Geometry: see drawing. Coordinates: mm, zero at the bounding-box minimum. A direction names the side the tool comes from. Round coordinates to 2 decimals unless told otherwise and drop trailing zeros. Write each loop counter-clockwise with the first axis right and the second up, starting at its lowest first coordinate (ties: lowest second). Pieces come first, ordered by that corner, then holes. Notation, with made-up numbers: (49.5, 26.5) -> (56.5, 26.5) arc R17 ccw to (56.5, 45.5) -> close; hole circle Ø4 at (0.25, 43). An arc over 180 degrees is marked (long way). Write item = value, one per line.
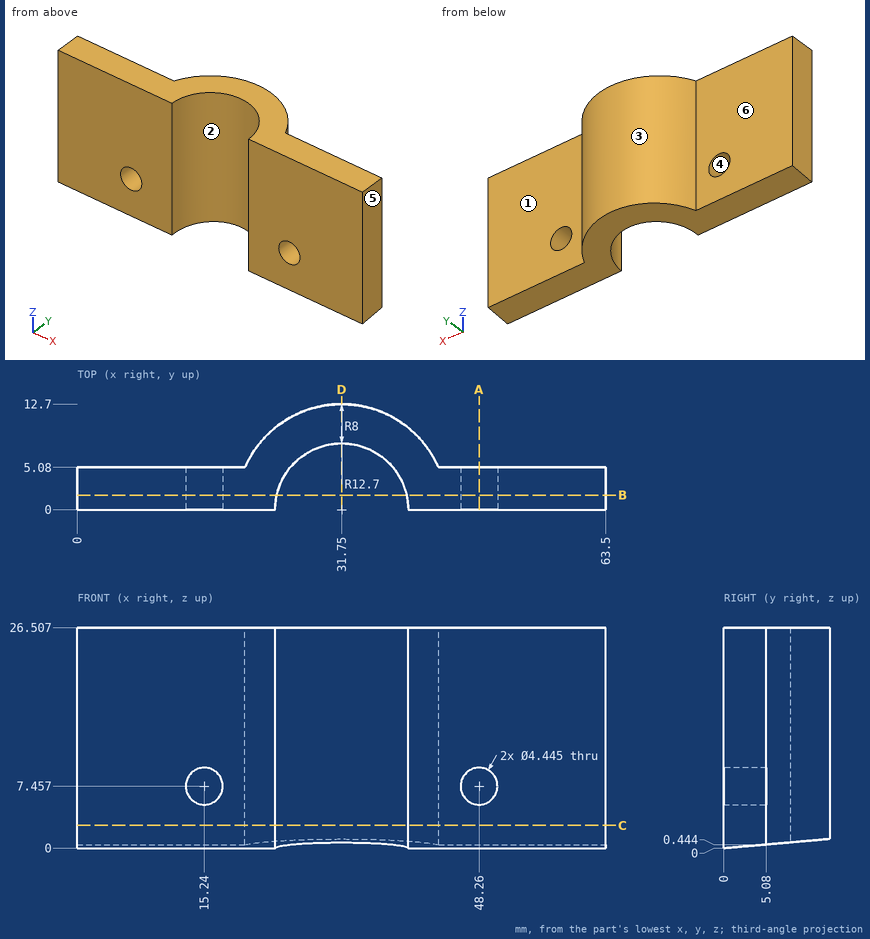
1) Cut plane D-D (x = 31.75). Return the cut outline in (y, z), and give its area (3 significant figures).
Solutions:
outline = (8, 0.7) -> (12.7, 1.11) -> (12.7, 26.51) -> (8, 26.51) -> close
area = 120 mm^2
2) Cut plane B-B (y = 1.75). Return the cut outline in (x, z) (1 decimal).
Solutions:
outline = (0, 0.2) -> (23.9, 0.2) -> (23.9, 26.5) -> (0, 26.5) -> close; (39.6, 0.2) -> (63.5, 0.2) -> (63.5, 26.5) -> (39.6, 26.5) -> close; hole circle Ø4.4 at (15.2, 7.5); hole circle Ø4.4 at (48.3, 7.5)
3) Access query for the marked faces 5 and 6. Directions: +Z, -Z, +X, -X, +Y, -Y. A direction counts if a zero-diameter tool reaches every point of the face in a straight line with its end or side. Return the directions, or none.
Solutions:
face_5 = +Z, -Z, +X, +Y, -Y
face_6 = +Z, -Z, -X, +Y
4) Cut plane C-C (z = 2.75). Return the cut outline in (x, y), and give its area (3 significant figures).
Solutions:
outline = (0, 0) -> (23.75, 0) arc R8 cw to (39.75, 0) -> (63.5, 0) -> (63.5, 5.08) -> (43.39, 5.08) arc R12.7 ccw to (20.11, 5.08) -> (0, 5.08) -> close
area = 350 mm^2
5) Cut plane A-A (x = 48.26). Return the cut outline in (y, z) (1 decimal).
Solutions:
outline = (0, 0) -> (5.1, 0.4) -> (5.1, 5.2) -> (0, 5.2) -> close; (0, 9.7) -> (5.1, 9.7) -> (5.1, 26.5) -> (0, 26.5) -> close
6) Draft query along X for the marked faces 1, 2, 3 and 4. Return one class per face: +X half, -X half, draft (parallel to the pull), parting line (faces both ways), or undercut.
Solutions:
face_1 = draft
face_2 = undercut
face_3 = parting line
face_4 = undercut
7) First-contact query: P1, Ø10, axis at x = 53.5, z = 16.5, coming from the +Y side; P2, Ø4, axis at x = 48.26, z = 7.46, coming from the -Y side; P3, Ø6, axis at y = 9.5, z = 10, coming from the -X side. Flat tips, straight axial feed; report the tip coordinate or a pass-through.
Solutions:
P1 = 5.08
P2 = through
P3 = 20.84
8) Line query: L1, parallel to X at y = 1.5, z = 7.75; L2, parallel to Y at x = 53.5, z = 17.75; L3, parallel to X at y = 2.75, z = 4.5. Output: solid intervals per line, ascending. Write a range as from..to.
Solutions:
L1 = 0..13.04, 17.44..23.89, 39.61..46.06, 50.46..63.5
L2 = 0..5.08
L3 = 0..24.24, 39.26..63.5
